Autodesk Inventor part; units mm, degrees
ref_plane "YZ Plane" through (0, 0, 0) normal (1, 0, 0) x (0, 1, 0)
ref_plane "XZ Plane" through (0, 0, 0) normal (0, 1, 0) x (-1, 0, 0)
ref_plane "XY Plane" through (0, 0, 0) normal (0, 0, 1) x (1, 0, 0)
sketch "Sketch1" plane through (0, 0, 0) normal (0, 1, 0) x (-1, 0, 0)
  line L0 (0, -20) -> (-30, -20)
  line L1 (-30, -20) -> (-30, 0)
  line L2 (-30, 0) -> (0, 0)
  line L3 (0, 0) -> (0, -20)
  dimension "d0" = 20
  dimension "d1" = 30
extrude "Extrusion1" add sketch "Sketch1" along normal blind 3
sketch "Sketch10" plane through (0, 3, 0) normal (0, 1, 0) x (1, 0, 0)
  circle A0 centre (5, 10) radius 1.6
  circle A1 centre (25, 10) radius 1.6
  line L0 (30, 20) -> (0, 20)
  line L1 (0, 0) -> (30, 0)
  line L2 (0, 20) -> (0, 0)
  line L3 (30, 0) -> (30, 20)
  line L4 (5, 10) -> (10, 10) construction
  line L5 (5, 8.4) -> (10, 8.4)
  line L6 (10, 11.6) -> (5, 11.6)
  arc A2 (5, 11.6) -> (5, 8.4) centre (5, 10) ccw
  arc A3 (10, 8.4) -> (10, 11.6) centre (10, 10) ccw
  line L7 (25, 10) -> (20, 10) construction
  line L8 (25, 8.4) -> (20, 8.4)
  line L9 (20, 11.6) -> (25, 11.6)
  arc A4 (25, 8.4) -> (25, 11.6) centre (25, 10) ccw
  arc A5 (20, 11.6) -> (20, 8.4) centre (20, 10) ccw
  point P0 (7.5, 10)
  point P1 (22.5, 10)
  dimension "d66" = 3.2
  dimension "d64" = 20
  dimension "d65" = 10
  dimension "d67" = 5
  dimension "d68" = 20
  dimension "d69" = 5
  dimension "d79" = 5
  dimension "d80" = 5
extrude "Extrusion6" cut sketch "Sketch10" against normal through all contours A0 | A0 L6 A3 L5 | A1 | A1 L8 A5 L9
fillet "Fillet5" radius 8 4 edges at (0, 1.5, 0) (0, 1.5, -20) (30, 1.5, -20) (30, 1.5, 0)
chamfer "Chamfer5" distance 2 angle 45 2 edges at (3.4, 3, -10) (26.6, 3, -10)
chamfer "Chamfer6" distance 2 angle 45 8 edges at (15, 3, 0) (27.6569, 3, -2.3431) (30, 3, -10) (27.6569, 3, -17.6569) (15, 3, -20) (2.3431, 3, -17.6569) (0, 3, -10) (2.3431, 3, -2.3431)
equation "\"d65\" = 0.5 * d64"
properties part number "synth-straight-bracket"
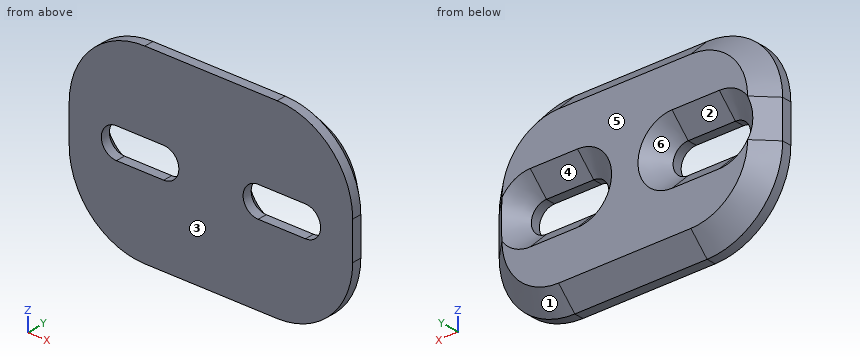
For this review, take the finished solid that the model builds, in its own axes (mm). Face numbers are marked on the shaded views. A direction names the side the tool comes from. Coordinates: 2 decimals unless noted, no trailing zeros. Order: outer loops, then holes, each group sorted by start corner. A loop starts at its lowest first (then second) coordinate and runs counter-clockwise, first axis right, second up. Notation, with made-up numbers: (11.5, 48.5) - (16.5, 48.5) arc R18 ccw to (16.5, 70.5) - close; hole circle Ø9 at (65.25, 52.25). An arc over 180 degrees is marked (long way). Answer as CSV lines item,"result". Start each with the question number.
1) Draft analysis for pull direction X (two halves, no side actions). For the marked faces 1, 2, 3 and 4, state which applies: +X half, -X half, draft (parallel to the pull), parting line (faces both ways), or undercut.
2) Add section C-C (y = 0.65). State the section outline as (x, z) points.
3) Add section A-A (x = 9.5). State the section outline as (y, z) points.
4) To check wall thickness, follow line 1 along X through (y, z) = (0.5, -9); line 2 along X through (y, z) = (1.7, -11.25); line 3 along Z through (x, y) = (7.25, 1.9). State the ranges of each line that lie inside material, in increasing order. Write a range as [from, to].
5) Insertion check: P1, Ø0.8, axis at x = 22.5, y = 0.5, coming from the -Z side; P2, Ø0.5, axis at x = 23, y = 0.5, coming from the +Z side. Each pin has a flat end and moves straight along its axis. Give the tip position at first contact, or say it passes through.
6) Add section D-D (y = 2.4). State the section outline as (x, z) points, then the cut area to 3 significant figures.
7) Add section B-B (z = -10). State the section outline as (x, y) points.
8) Machinability: for the marked faces 5 and 6, which of the approach directions +Z, -Z, +X, -X, +Y, -Y give a long, thin tool a straight path to every point of the face, cutting with its end or side? Answer none if there is none.
Result:
1,face 1,"+X half"
1,face 2,"undercut"
1,face 3,"draft"
1,face 4,"undercut"
2,outline,"(0, -12) arc R8 ccw to (8, -20) - (22, -20) arc R8 ccw to (30, -12) - (30, -8) arc R8 ccw to (22, 0) - (8, 0) arc R8 ccw to (0, -8) - close; hole (5, -11.6) - (10, -11.6) arc R1.6 ccw to (10, -8.4) - (5, -8.4) arc R1.6 ccw to start; hole (20, -11.6) - (25, -11.6) arc R1.6 ccw to (25, -8.4) - (20, -8.4) arc R1.6 ccw to start"
3,outline,"(0, -20) - (1, -20) - (3, -18) - (3, -13.6) - (1, -11.6) - (0, -11.6) - close; (0, -8.4) - (1, -8.4) - (3, -6.4) - (3, -2) - (1, 0) - (0, 0) - close"
4,line 1,"[0, 3.75], [11.25, 18.75], [26.25, 30]"
4,line 2,"[0.7, 3.07], [11.93, 18.07], [26.93, 29.3]"
4,line 3,"[-19.06, -12.5], [-7.5, -0.94]"
5,P1,"z = -20"
5,P2,"z = -0.04"
6,outline,"(1.4, -12) arc R6.6 ccw to (8, -18.6) - (22, -18.6) arc R6.6 ccw to (28.6, -12) - (28.6, -8) arc R6.6 ccw to (22, -1.4) - (8, -1.4) arc R6.6 ccw to (1.4, -8) - close; hole (5, -13) - (10, -13) arc R3 ccw to (10, -7) - (5, -7) arc R3 ccw to start; hole (20, -13) - (25, -13) arc R3 ccw to (25, -7) - (20, -7) arc R3 ccw to start"
6,area,"314 mm^2"
7,outline,"(0, 0) - (3.4, 0) - (3.4, 1) - (1.7, 2.7) - (0, 1) - close; (11.6, 0) - (18.4, 0) - (18.4, 1) - (16.4, 3) - (13.6, 3) - (11.6, 1) - close; (26.6, 0) - (30, 0) - (30, 1) - (28.3, 2.7) - (26.6, 1) - close"
8,face 5,"+Z, -Z, +X, -X, +Y"
8,face 6,"+Y"
